Source: three-view drawing plus pictorial views. Frame: mm from the lowest corner of the part. A direction names the side the tool comes from. Give positions to 0.01 mm unless a question says otherwise; leave off trailing zeros. Loops run counter-clockwise (first coordinate to the right, second up) from the corner with the lowest first, then second, coordinate; pieces in that order, holes last. Notation, with made-up numbers: (16.5, -1.75) - (55.5, -1.75) arc R34 ccw to (55.5, 36.25) - close; hole circle Ø2 at (60, 5.5). An arc over 180 degrees is marked (long way). Answer as a JSON object with one key per item and string values. Group by question number.
(1) Access query for the marked faces 1 and 2. Directions: +Z, -Z, +X, -X, +Y, -Y. A direction counts if a zero-diameter tool reaches every point of the face in a straight line with its end or side. Return the directions, or none.
(2) Pin query (flat end, axial travel): P1, Ø1.8, axis at x = 2.3, y = 2.3, coming from the +Z side. Return the tip coordinate at first contact, or that it passes through.
(3) Mould query, pull axis X, two halves, no side actions, for the marked faces 3, 4, 5 and 6. Classes: +X half, -X half, draft (parallel to the pull), parting line (faces both ways), or undercut.
(4) Section query B-B (x = 10.1). Return loops of the section in (y, z), plus the area to 3 significant figures.
(5) Section query A-A (z = 9.75). Return loops of the section in (x, y).
(6) Material intervals for L1, parallel to Y at x = 10.1, z = 0.6; L2, parallel to X at y = 17.75, z = 8.25; L3, parallel to Y at x = 10.1, z = 6.5, sorted ascending.
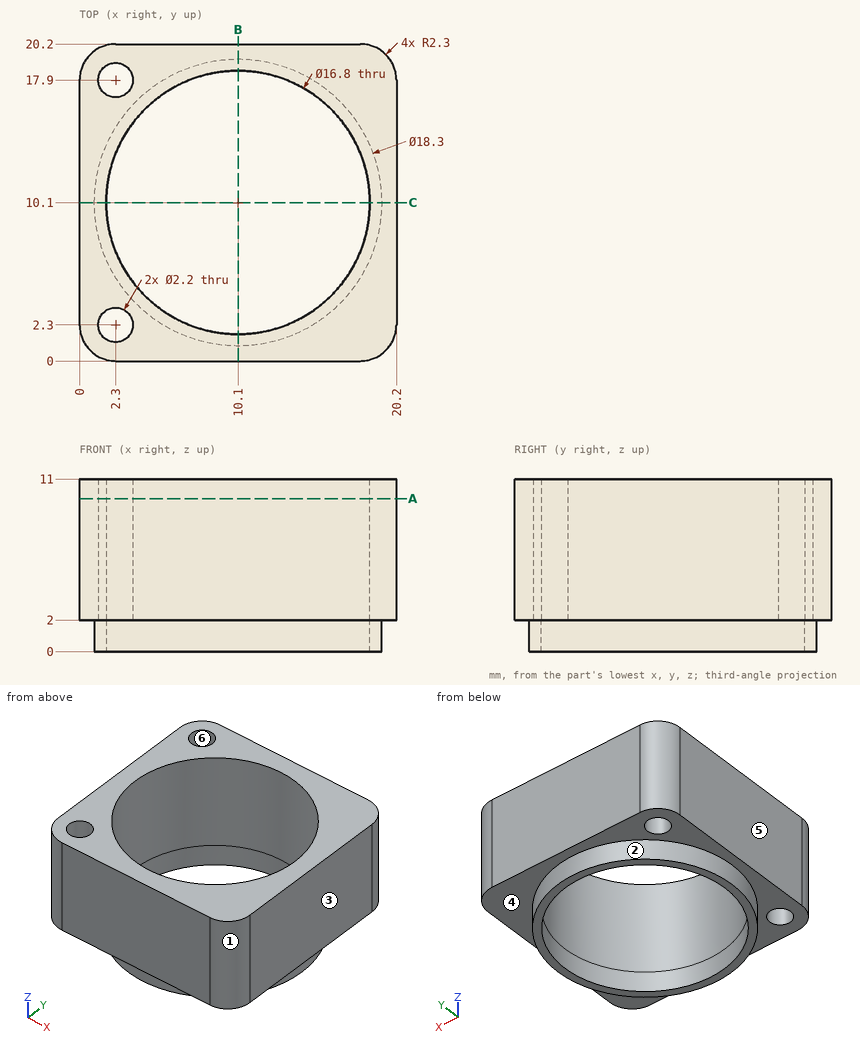
Recorded:
{
 "1": {"face 1": "+Z, -Z, +X, -Y", "face 2": "-Z"},
 "2": {"P1": "passes through"},
 "3": {"face 3": "+X half", "face 4": "draft", "face 5": "-X half", "face 6": "undercut"},
 "4": {"outline": "(0, 2) - (0.95, 2) - (0.95, 0) - (1.7, 0) - (1.7, 11) - (0, 11) - close; (18.5, 0) - (19.25, 0) - (19.25, 2) - (20.2, 2) - (20.2, 11) - (18.5, 11) - close", "area": "33.6 mm^2"},
 "5": {"outline": "(0, 2.3) arc R2.3 ccw to (2.3, 0) - (17.9, 0) arc R2.3 ccw to (20.2, 2.3) - (20.2, 17.9) arc R2.3 ccw to (17.9, 20.2) - (2.3, 20.2) arc R2.3 ccw to (0, 17.9) - close; hole circle Ø2.2 at (2.3, 2.3); hole circle Ø2.2 at (2.3, 17.9); hole circle Ø16.8 at (10.1, 10.1)"},
 "6": {"L1": "y = 0.95 to 1.7, 18.5 to 19.25", "L2": "x = 0 to 1.21, 3.39 to 6.63, 13.57 to 20.2", "L3": "y = 0 to 1.7, 18.5 to 20.2"}
}
